Can you work these out from the model? Positions are in its coordinate system, mm. A direction names the side the tool comes from. Give positions to 0.01 mm unless a question says otherwise; leave off trailing zeros. Loops run counter-clockwise (first coordinate to the right, second up) from the corner with the lowest first, then second, coordinate; pieces in that order, holes last.
from build123d import *

# Parameters (mm, degrees)
AUFSATZ_LINEAR_AUSTRAGEN1_DEPTH                      = 2
SKIZZE2_W                                            = 123
SKIZZE2_H                                            = 2
AUFSATZ_LINEAR_AUSTRAGEN2_DEPTH                      = 30
VERRUNDUNG1_R                                        = 2
VERRUNDUNG2_R                                        = 4
SKIZZE3_R                                            = 3
SCHNITT_LINEAR_AUSTRAGEN1_DEPTH                      = 152.345576266
FORMSENKUNG_F_R_M4_SENKSCHRAUBE_MIT_INNE_D           = 4.5
FORMSENKUNG_F_R_M4_SENKSCHRAUBE_MIT_INNE_DEPTH       = 11.94
FORMSENKUNG_F_R_M4_SENKSCHRAUBE_MIT_INNE_CSINK_D     = 9.18
FORMSENKUNG_F_R_M4_SENKSCHRAUBE_MIT_INNE_CSINK_ANGLE = 90
FORMSENKUNG_F_R_M4_SENKSCHRAUBE_MIT_INNE_TIP         = 1.351936393
SKIZZE7_R                                            = 1.95
SKIZZE7_R_2                                          = 31
SCHNITT_LINEAR_AUSTRAGEN2_DEPTH                      = 106.295533596


with BuildPart() as part:
    # Skizze1 → Aufsatz-Linear austragen1 (new body)
    with BuildSketch(Plane.XY):
        Polygon((-69.023447297, -46.645824625), (-48.023447297, -46.645824625), (-48.023447297, -66.645824625), (74.976552703, -66.645824625), (74.976552703, 61.354175375), (-69.023447297, 61.354175375), align=None)
    extrude(amount=AUFSATZ_LINEAR_AUSTRAGEN1_DEPTH)

    # Skizze2 → Aufsatz-Linear austragen2 (add)
    with BuildSketch(Plane(origin=(0, 0, 0), x_dir=(-1, 0, 0), z_dir=(0, 0, -1))):
        with Locations((-13.476552703, -65.645824625)):
            Rectangle(SKIZZE2_W, SKIZZE2_H)
    extrude(amount=AUFSATZ_LINEAR_AUSTRAGEN2_DEPTH)

    # Verrundung1
    verrundung1_edges = [part.edges().sort_by_distance(p)[0] for p in [
        (13.476552703, -64.645824625, 0),
    ]]
    fillet(verrundung1_edges, radius=VERRUNDUNG1_R)

    # Verrundung2
    verrundung2_edges = [part.edges().sort_by_distance(p)[0] for p in [
        (13.476552703, -66.645824625, 2),
    ]]
    fillet(verrundung2_edges, radius=VERRUNDUNG2_R)

    # Skizze3 → Schnitt-Linear austragen1 (cut, through all)
    with BuildSketch(Plane.XZ.offset(66.645824625)):
        with Locations((-33.023447297, -16)):
            Circle(SKIZZE3_R)
        with Locations((59.976552703, -16)):
            Circle(SKIZZE3_R)
    extrude(amount=-SCHNITT_LINEAR_AUSTRAGEN1_DEPTH, mode=Mode.SUBTRACT)

    # Formsenkung für M4 Senkschraube mit Innensechskant1
    with Locations(Plane.XY.offset(2)):
        with Locations((-59.023447297, -31.645824625), (-59.023447297, 46.354175375)):
            CounterSinkHole(FORMSENKUNG_F_R_M4_SENKSCHRAUBE_MIT_INNE_D / 2, FORMSENKUNG_F_R_M4_SENKSCHRAUBE_MIT_INNE_CSINK_D / 2, depth=FORMSENKUNG_F_R_M4_SENKSCHRAUBE_MIT_INNE_DEPTH, counter_sink_angle=FORMSENKUNG_F_R_M4_SENKSCHRAUBE_MIT_INNE_CSINK_ANGLE)
            with Locations((0, 0, -(FORMSENKUNG_F_R_M4_SENKSCHRAUBE_MIT_INNE_DEPTH + FORMSENKUNG_F_R_M4_SENKSCHRAUBE_MIT_INNE_TIP / 2))):  # 118° drill point
                Cone(0, FORMSENKUNG_F_R_M4_SENKSCHRAUBE_MIT_INNE_D / 2, FORMSENKUNG_F_R_M4_SENKSCHRAUBE_MIT_INNE_TIP, mode=Mode.SUBTRACT)

    # Skizze7 → Schnitt-Linear austragen2 (cut, through all)
    with BuildSketch(Plane.XY.offset(2)):
        with Locations((17.976552703, 41.354175375)):
            Circle(SKIZZE7_R)
        with Locations((49.442804466, 28.320427137)):
            Circle(SKIZZE7_R)
        with Locations((49.442804466, -34.612076388)):
            Circle(SKIZZE7_R)
        with Locations((17.976552703, -47.645824625)):
            Circle(SKIZZE7_R)
        with Locations((-13.489699059, -34.612076388)):
            Circle(SKIZZE7_R)
        with Locations((-13.489699059, 28.320427137)):
            Circle(SKIZZE7_R)
        with Locations((17.976552703, -3.145824625)):
            Circle(SKIZZE7_R_2)
        with Locations((-24.523447297, -3.145824625)):
            Circle(SKIZZE7_R)
        with Locations((60.476552703, -3.145824625)):
            Circle(SKIZZE7_R)
        with BuildLine():
            Line((-61.881657041, -16.935182234), (-61.881657041, 32.354175375))
            ThreePointArc((-61.881657041, 32.354175375), (-59.023447297, 35.212385119), (-56.165237552, 32.354175375))
            Line((-56.165237552, 32.354175375), (-56.165237552, -16.935182234))
            ThreePointArc((-56.165237552, -16.935182234), (-59.023447297, -19.793391979), (-61.881657041, -16.935182234))
        make_face()
    extrude(amount=-SCHNITT_LINEAR_AUSTRAGEN2_DEPTH, mode=Mode.SUBTRACT)


solid = part.part
(1) Thinking about a two-plate mould opening in Y: for faces 3 (the cylindrical face through (-33.67, -65.66, -18.93)), 4 (the flat face through (14, -66.646, -16)), 5 (the cylindrical face through (-22.663, -2.56, 1.014)), which applies, pulls with the +Y half, pulls with the -Y half, needs draft (parallel to the pull), parting line crosses it, or undercut?
Returned:
face 3: needs draft
face 4: pulls with the -Y half
face 5: undercut
(2) Suppose I cut it at A-A on z = -16. List the corners of the cut face in (x, y) for me, plus the area to 3 significant figures.
Returned:
outline: (-48.02, -66.65) - (-36.02, -66.65) - (-36.02, -64.65) - (-48.02, -64.65) - close; (-30.02, -66.65) - (56.98, -66.65) - (56.98, -64.65) - (-30.02, -64.65) - close; (62.98, -66.65) - (74.98, -66.65) - (74.98, -64.65) - (62.98, -64.65) - close
area: 222 mm2
(3) Which directions (+Z, -Z, +X, -X, +Y, -Y) give clear straight access to the entire face, cutting with the end or side of a thin tool? Please do faces 1 (the flat face through (-14, 0, 0)), 2 (the cylindrical face through (14.3, -65.5, 0.8)).
Returned:
face 1: -Z, +X, -X, +Y
face 2: +Z, +X, -X, -Y
(4) Suppose I cut it at D-D on z = -7.5. List the corners of the cut face in (x, y) for me.
Returned:
outline: (-48.02, -66.65) - (74.98, -66.65) - (74.98, -64.65) - (-48.02, -64.65) - close
(5) Please list where these lines run through material, in increasing order: probe 1 along Z at (x, y) = (-41, -28); probe 2 along Y at (x, z) = (-30.5, -9.5); probe 3 along X at (y, z) = (-54, 0.5).
Returned:
probe 1: z = 0 to 2
probe 2: y = -66.65 to -64.65
probe 3: x = -48.02 to 74.98
(6) Suppose I cut it at B-B on x = -43.5. List the corners of the cut face in (y, z) for me.
Returned:
outline: (-66.65, -30) - (-64.65, -30) - (-64.65, -2) arc R2 cw to (-62.65, 0) - (61.35, 0) - (61.35, 2) - (-62.65, 2) arc R4 ccw to (-66.65, -2) - close
(7) Suppose I cut it at C-C on x = 41.5. List the corners of the cut face in (y, z) for me.
Returned:
outline: (-66.65, -30) - (-64.65, -30) - (-64.65, -2) arc R2 cw to (-62.65, 0) - (-23.34, 0) - (-23.34, 2) - (-62.65, 2) arc R4 ccw to (-66.65, -2) - close; (17.04, 0) - (61.35, 0) - (61.35, 2) - (17.04, 2) - close
(8) Will these pins go through, and if not, where does the flat tip stop? P1, Ø1.6, axis at x = -57.5, z = 0.5, coming from the -Y side; P2, Ø4, axis at x = -38.5, y = 3.5, coming from the -Z side; P3, Ø10, axis at x = -10, z = -7, coming from the +Y side.
Returned:
P1: stops at y = -46.65
P2: stops at z = 0
P3: stops at y = -64.65
